```python
from build123d import *

# Parameters (mm, degrees)
BOSS_EXTRUDE1_DEPTH = 457.2
CUT_EXTRUDE1_REACH  = 462.55
SKETCH2_R           = 3.175
CUT_EXTRUDE2_DEPTH  = 461.714271539
CUT_EXTRUDE3_DEPTH  = 461.714271539


with BuildPart() as part:
    # Sketch1 → Boss-Extrude1 (new body)
    with BuildSketch(Plane.XY):
        Polygon((3.175, 3.175), (3.175, 25.4), (0, 25.4), (0, 0), (50.8, 0), (50.8, 25.4), (47.625, 25.4), (47.625, 3.175), align=None)
    extrude(amount=BOSS_EXTRUDE1_DEPTH)

    # Sketch2 → Cut-Extrude1 (cut, up to next)
    with BuildSketch(Plane(origin=(0, 3.175, 0), x_dir=(1, 0, 0), z_dir=(0, 1, 0)), mode=Mode.PRIVATE) as cut_extrude1_sk1:
        with Locations(Location((12.384908578, -132.81875466, 0), (0, 0, 270))):
            Circle(SKETCH2_R)
    cut_extrude1_tool1 = extrude(cut_extrude1_sk1.sketch, amount=-CUT_EXTRUDE1_REACH, mode=Mode.PRIVATE) & part.part
    add(cut_extrude1_tool1.solids().sort_by_distance((12.384909, 3.175, 132.818755))[0], mode=Mode.SUBTRACT)

    # Sketch3 → Cut-Extrude2 (cut, through all)
    with BuildSketch(Plane.ZY):
        Polygon((0, 25.4), (21.313130632, 0), (0, 0), align=None)
    extrude(amount=-CUT_EXTRUDE2_DEPTH, mode=Mode.SUBTRACT)

    # Sketch4 → Cut-Extrude3 (cut, through all)
    with BuildSketch(Plane(origin=(50.8, 0, 0), x_dir=(0, 0, -1), z_dir=(1, 0, 0))):
        Polygon((-352.886582122, 0), (-331.57345149, 25.4), (-457.2, 25.4), (-457.2, 0), align=None)
    extrude(amount=-CUT_EXTRUDE3_DEPTH, mode=Mode.SUBTRACT)


solid = part.part
```
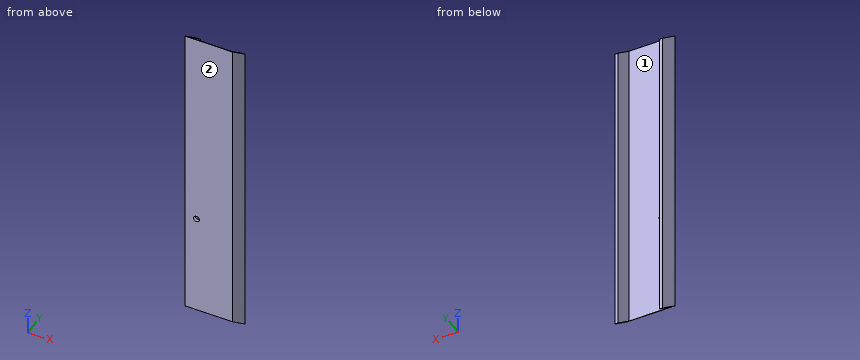
Read the model definition and answer for the solid it produces. Units are mm, in the model's axes. Face numbers are marked on the shaded views. Coordinates: 2 decimals unless noted, no trailing zeros. Write each loop counter-clockwise with the first axis right and the second up, starting at its lowest first coordinate (ties: lowest second). Pieces come first, ordered by that corner, then holes. Notation, with made-up numbers: (58.5, -10) -> (65.5, -10) arc R32 ccw to (65.5, 17) -> close; hole circle Ø2 at (77, 30.5). An arc over 180 degrees is marked (long way). Write item = value, one per line.
(1) Given pin 1 Ø12 at (x, z) = (25.5, 181) entering from +Y (3 decimals); pin 2 Ø5 at (x, z) = (12.38, 132.82) entering from -Y, each flat-ended and moving along its own axis, determine where each tip first touches the part or whether it passes through.
From the geometry:
pin_1 = 3.175
pin_2 = through
(2) Section B-B on z = 193 is taken. Write down the section's boundary in (x, y) (3 decimals), plus the area to 3 significant figures.
From the geometry:
outline = (0, 0) -> (50.8, 0) -> (50.8, 25.4) -> (47.625, 25.4) -> (47.625, 3.175) -> (3.175, 3.175) -> (3.175, 25.4) -> (0, 25.4) -> close
area = 302 mm2
(3) Straight lines are drawn through the part: L1, parallel to X at y = 17.5, z = 222 (3 decimals); L2, parallel to Y at x = 26, z = 265.5 (3 decimals); L3, parallel to Z at x = 27, y = 1.75. For each, find the intervals that lie inside material, in ascending order. Write a range as from..to.
From the geometry:
L1 = 0..3.175, 47.625..50.8
L2 = 0..3.175
L3 = 19.84..351.42
(4) For a pull along X with two mould halves and no side action, classify the marked faces 1 and 2 as +X half, -X half, draft (parallel to the pull), parting line (faces both ways), or undercut.
From the geometry:
face_1 = undercut
face_2 = draft
(5) Section A-A on y = 14.5 is taken. Write down the section's boundary in (x, z) (3 decimals).
From the geometry:
outline = (0, 9.146) -> (3.175, 9.146) -> (3.175, 340.72) -> (0, 340.72) -> close; (47.625, 9.146) -> (50.8, 9.146) -> (50.8, 340.72) -> (47.625, 340.72) -> close
(6) Section C-C on x = 21 is taken. Write down the section's boundary in (y, z) (3 decimals).
From the geometry:
outline = (0, 21.313) -> (3.175, 18.649) -> (3.175, 350.222) -> (0, 352.887) -> close
